from build123d import *

# Parameters (mm, degrees)
SKETCH001_W  = 2.6
SKETCH001_H  = 2.6
PAD_DEPTH    = 3.5
SKETCH_W     = 15
SKETCH_H     = 8
PAD001_DEPTH = 0.5
SKETCH002_W  = 4.9
SKETCH002_H  = 4.9
PAD002_DEPTH = 6


with BuildPart() as pad:
    # Sketch001 → Pad (new body)
    with BuildSketch(Plane.XY):
        with Locations((7.5, 4)):
            Rectangle(SKETCH001_W, SKETCH001_H)
    extrude(amount=PAD_DEPTH)


with BuildPart() as pad001:
    # Sketch → Pad001 (new body)
    with BuildSketch(Plane.XY):
        with Locations((7.5, 4)):
            Rectangle(SKETCH_W, SKETCH_H)
    extrude(amount=PAD001_DEPTH)


with BuildPart() as cut:
    # Sketch002 → Pad002 (new body)
    with BuildSketch(Plane.XY):
        with Locations((7.55, 4.05)):
            Rectangle(SKETCH002_W, SKETCH002_H)
    extrude(amount=PAD002_DEPTH)

    # Fusion: union Pad001
    add(pad001.part)

    # Cut: cut Pad
    add(pad.part, mode=Mode.SUBTRACT)


solid = cut.part
The model under review builds one solid part; all positions refer to its coordinate system, in mm. A direction names the side the tool comes from. Round coordinates to 2 decimals unless told otherwise and drop trailing zeros. Order: outer loops, then holes, each group sorted by start corner. A loop starts at its lowest first (then second) coordinate and runs counter-clockwise, first axis right, second up. Notation, with made-up numbers: (13.25, 4.5) - (45.25, 4.5) arc R21 ccw to (45.25, 8.5) - close; hole circle Ø2 at (86.25, -14.75). An arc over 180 degrees is marked (long way). Use one line per item in the form item = value.
Q1. Add section D-D on x = 8. Give the boundary of the cut face in (y, z).
Response values:
outline = (0, 0) - (2.7, 0) - (2.7, 3.5) - (5.3, 3.5) - (5.3, 0) - (8, 0) - (8, 0.5) - (6.5, 0.5) - (6.5, 6) - (1.6, 6) - (1.6, 0.5) - (0, 0.5) - close
Q2. Clearance check with flat-ended pins moving along their axes: P1, Ø2, axis at y = 3.5, z = 2.5, coming from the -X side; P2, Ø0.8, axis at x = 7.5, z = 1.5, coming from the +Y side; P3, Ø3, axis at x = 9, z = 3.5, coming from the -Y side. State where each tip first meets the part, or that it passes through.
Response values:
P1 = 5.1
P2 = 6.5
P3 = 1.6
Q3. To check wall thickness, follow line 1 (Y direction, x = 7.5, z = 0.45); line 2 (Y direction, x = 6.25, z = 3.25); line 3 (X direction, y = 2.75, z = 1.3). State the ranges of each line that lie inside material, in increasing order.
Response values:
line_1 = 0 to 2.7, 5.3 to 8
line_2 = 1.6 to 2.7, 5.3 to 6.5
line_3 = 5.1 to 6.2, 8.8 to 10
Q4. Add section A-A on z = 0.9. Give the boundary of the cut face in (x, y).
Response values:
outline = (5.1, 1.6) - (10, 1.6) - (10, 6.5) - (5.1, 6.5) - close; hole (6.2, 2.7) - (8.8, 2.7) - (8.8, 5.3) - (6.2, 5.3) - close
Q5. Add section C-C on y = 3.5. Give the boundary of the cut face in (x, z).
Response values:
outline = (0, 0) - (6.2, 0) - (6.2, 3.5) - (8.8, 3.5) - (8.8, 0) - (15, 0) - (15, 0.5) - (10, 0.5) - (10, 6) - (5.1, 6) - (5.1, 0.5) - (0, 0.5) - close
Q6. Tool access review of faces 4 (the flat face through (8, 6.5, 3)), 5 (the flat face through (8.8, 4, 2)), 6 (the flat face through (10, 4, 3)): name each direction out of +Z, -Z, +X, -X, +Y, -Y from which nothing blocks a thin tool from reaching the whole face with its end or side.
Response values:
face_4 = +Z, +X, -X, +Y
face_5 = -Z
face_6 = +Z, +X, +Y, -Y
Q7. Mouldability with a two-part tool opening along Y and no side actions: class faces 1 (the flat face through (7, 1, 0.5)), 2 (the flat face through (7, 4, 3.5)), 3 (the flat face through (8, 1.6, 3)) as pulls with the +Y half, pulls with the -Y half, needs draft (parallel to the pull), parting line crosses it, or undercut.
Response values:
face_1 = needs draft
face_2 = undercut
face_3 = pulls with the -Y half
Q8. Add section B-B on x = 5.25. Give the boundary of the cut face in (y, z).
Response values:
outline = (0, 0) - (8, 0) - (8, 0.5) - (6.5, 0.5) - (6.5, 6) - (1.6, 6) - (1.6, 0.5) - (0, 0.5) - close
